Geometry: see drawing. Coordinates: mm, zero at the bounding-box minimum. A direction names the side the tool comes from. Give positions to 0.01 mm unless a question says otherwise; leave off trailing zeros. Order: outer loops, then holes, each group sorted by start corner. A loop starts at its lowest first (then second) coordinate and runs counter-clockwise, first axis right, second up. Notation, with made-up numbers: (80.25, 59) - (134.25, 59) arc R9 cw to (134.25, 64) - close; hole circle Ø2 at (72.25, 51.5). An arc over 180 degrees is marked (long way). Write each question's results on one line, items separated by ' | '. Start each with the question number.
Item 1: Section D-D on x = 48. Output: boundary loops of the cut face in (y, z).
Item 2: Section A-A on y = 62.5. Output: boundary loops of the cut face in (x, z).
Item 3: Line query: line 1 along Y through (x, z) = (28.5, 12.5); line 2 along Y through (x, z) = (50, 21) (1 decimal); line 3 along X through (y, z) = (50, 7.5). Output: solid intervals per line, ascending.
Item 4: Set-up query: the marked faces 4, 5, 6, 7 and 8. Return all of +Z, -Z, +X, -X, +Y, -Y with unobstructed straight access to the full face (end or side cutting, diameter ignored); none if empty.
Item 5: Mould query, pull axis X, two halves, no side actions, for the marked faces 1, 2 and 3. Classes: released by +X, released by -X, zero draft, split by the parting line, or undercut.
Item 6: Section B-B on x = 90. Output: boundary loops of the cut face in (y, z).
Item 7: Contact query for flat-ended pins moving along their axis: pin 1 Ø12 at (y, z) = (8, 4) entering from +X (1 decimal); pin 2 Ø5 at (y, z) = (17.5, 19.5) entering from -X (1 decimal); pin 3 Ø1.8 at (x, y) = (49, 8.5) entering from -Z; pin 4 Ø4 at (x, z) = (7.87, 11) entering from +Y. Output: stop coordinate, or through.
Item 8: Section C-C on y = 13.5. Output: boundary loops of the cut face in (x, z).
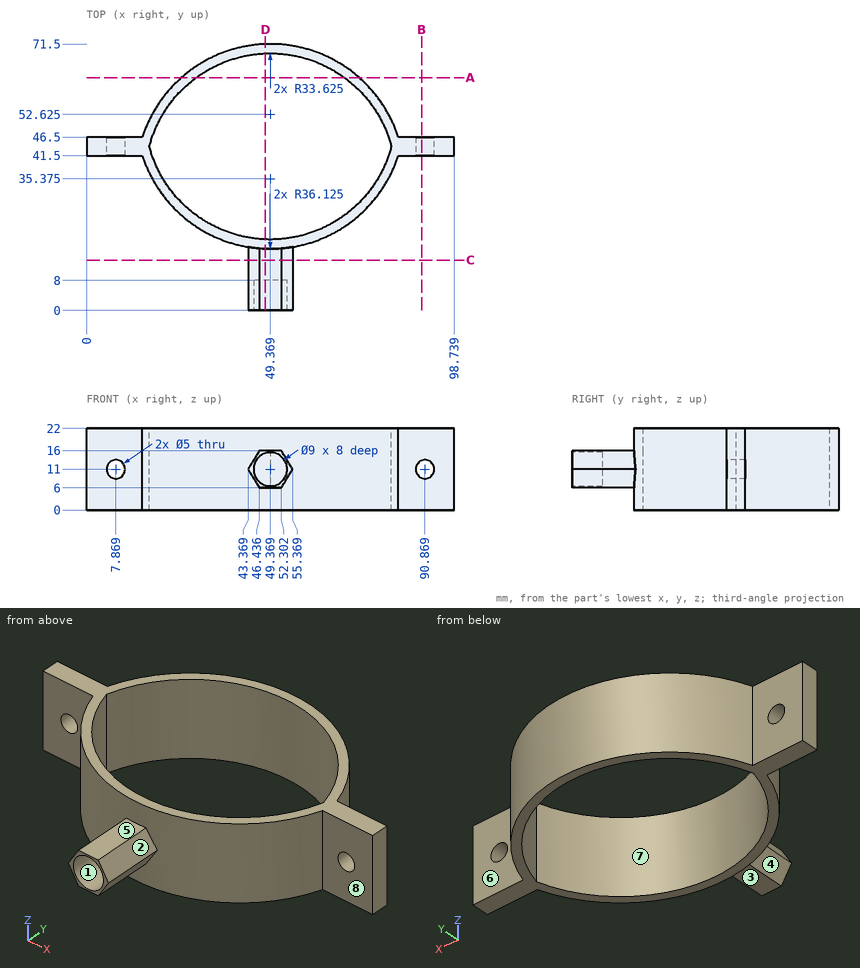
Evaluation:
1) outline: (0, 6) - (16.53, 6) - (16.53, 0) - (19.03, 0) - (19.03, 22) - (16.53, 22) - (16.53, 16) - (0, 16) - (0, 15.29) - (8, 15.29) - (8, 6.71) - (0, 6.71) - close; (68.97, 0) - (71.47, 0) - (71.47, 22) - (68.97, 22) - close
2) outline: (25.51, 0) - (29.5, 0) - (29.5, 22) - (25.51, 22) - close; (69.24, 0) - (73.23, 0) - (73.23, 22) - (69.24, 22) - close
3) line 1: y = 23.14 to 26.26, 61.74 to 64.86 | line 2: y = 16.5 to 19, 69 to 71.5 | line 3: x = 16.34 to 19.09, 79.65 to 82.4
4) face 4: -Z, -X, -Y | face 5: +Z, +X, -X, -Y | face 6: +Z, -Z, +X, +Y | face 7: +Z, -Z | face 8: +Z, -Z, +X, -Y
5) face 1: undercut | face 2: released by +X | face 3: zero draft
6) outline: (41.5, 0) - (46.5, 0) - (46.5, 8.66) - (41.5, 8.66) - close; (41.5, 13.34) - (46.5, 13.34) - (46.5, 22) - (41.5, 22) - close
7) pin 1: stops at x = 54.8 | pin 2: stops at x = 33.9 | pin 3: stops at z = 6 | pin 4: passes through
8) outline: (43.37, 11) - (46.44, 6) - (52.3, 6) - (55.37, 11) - (52.3, 16) - (46.44, 16) - close
